Geometry check sheet. Reference: the model listing, model coordinates, mm. A direction names the side the tool comes from. Give positions to 0.01 mm unless a question says otherwise; leave off trailing zeros. Write each loop counter-clockwise with the first axis right and the second up, starting at its lowest first coordinate (ties: lowest second). Pieces come first, ordered by that corner, then holes. Notation, with made-up numbers: (18.25, 16) - (34.25, 16) arc R29 ccw to (34.25, 54) - close; hole circle Ø8 at (58.25, -21.75). An arc over 180 degrees is marked (long way). One line per question, with ' | ' between items. Start each with the question number.
Q1. Set-up check for faces 1 (the face through (-118.726, 56.298, 153.37)), 2 (the face through (152.4, -95, -28)), 3 (the face through (101.6, -1, -64)): record each of +Z, -Z, +X, -X, +Y, -Y from which the full face is reachable in a straight line by a thin tool's end or side.
Q2. Section check B-B on z = -25.4. Record the boundary of the cut face in (x, y), and give its area (3 significant figures).
Q3. Section check C-C on x = 18. Record the boundary of the cut face in (y, z).
Q4. Release check for a two-part mould opening along X. For faces 4 (the face through (1.355, 120.166, -156.446)), 5 (the face through (-152.4, -46, -28)), 6 (the face through (118.726, 56.298, 153.37)), 7 (the face through (-23.622, -8.259, -62.594)) record: +X half, -X half, draft (parallel to the pull), parting line (faces both ways), or undercut.
Q5. Section check A-A on y = 0. Record the boundary of the cut face in (x, z).
Q6. Gauge pin test, flat ends, axial feed: P1, Ø2, axis at x = -110, z = -52, coming from the +Y side; P2, Ø5, axis at x = -121, y = -148, coming from the -Z side; P3, Ø1, axis at x = -95.5, y = 139.5, coming from the +Z side. Record the tip position at first contact, or that the pin passes through.
Q7. Thickness scan on L1, parallel to Y at x = 16.5, z = -26; L2, parallel to Z at x = 142.5, y = 0; L3, parallel to X at y = -202.5, z = -77.5. Record the ranges inside material, lowest first. Write a range as [from, to].
```python
from build123d import *

# Parameters (mm, degrees)
F3_R     = 38.1
F3_R_2   = 25.4
F4_DEPTH = 304.801
F5_R     = 88.9
F5_R_2   = 38.1
F6_DEPTH = 50.8


with BuildPart() as f1:
    # F0 (on Front) → F1 (revolve)
    with BuildSketch(Plane.XZ):
        with BuildLine():
            Line((-152.4, 0), (0, 0))
            Line((0, 0), (0, 152.4))
            Line((0, 152.4), (-96.757379, 152.4))
            ThreePointArc((-96.757379, 152.4), (-107.418768, 153.949285), (-116.478976, 159.778363))
            Line((-116.478976, 159.778363), (-152.4, 195.699387))
            Line((-152.4, 195.699387), (-152.4, 0))
        make_face()
    revolve(axis=Axis((-127.974883, 0, -25.4), (-1, 0, 0)))

    # F2: F1 across face


with BuildPart() as f1_1:
    add(f1.part)
    add(f1.part.mirror(Plane(origin=(0, 0, -25.4), x_dir=(0, 1, 0), z_dir=(1, 0, 0))))

    # F3 (on face) → F4 (cut, through all)
    with BuildSketch(Plane.YZ.offset(152.4)):
        with Locations((0, -25.4)):
            Circle(F3_R)
        with Locations((0, -25.4)):
            Circle(F3_R_2, mode=Mode.SUBTRACT)
    extrude(amount=-F4_DEPTH, mode=Mode.SUBTRACT)

    # F5 (on face) → F6 (cut)
    with BuildSketch(Plane.YZ.offset(152.4)):
        with Locations((0, -25.4)):
            Circle(F5_R)
        with Locations((0, -25.4)):
            Circle(F5_R_2, mode=Mode.SUBTRACT)
    extrude(amount=-F6_DEPTH, mode=Mode.SUBTRACT)


solid = f1_1.part
```
Working result:
1) face 1: none | face 2: +Z, -Z, +X, +Y, -Y | face 3: +X
2) outline: (-152.4, -221.1) - (-116.48, -185.18) arc R25.4 cw to (-96.76, -177.8) - (96.76, -177.8) arc R25.4 cw to (116.48, -185.18) - (152.4, -221.1) - (152.4, -88.9) - (101.6, -88.9) - (101.6, -38.1) - (-152.4, -38.1) - close; (-152.4, 38.1) - (101.6, 38.1) - (101.6, 88.9) - (152.4, 88.9) - (152.4, 221.1) - (116.48, 185.18) arc R25.4 cw to (96.76, 177.8) - (-96.76, 177.8) arc R25.4 cw to (-116.48, 185.18) - (-152.4, 221.1) - close | area: 83,800 mm2
3) outline: circle Ø355.6 at (0, -25.4); hole circle Ø76.2 at (0, -25.4)
4) face 4: undercut | face 5: -X half | face 6: undercut | face 7: draft
5) outline: (-152.4, -246.5) - (-116.48, -210.58) arc R25.4 cw to (-96.76, -203.2) - (96.76, -203.2) arc R25.4 cw to (116.48, -210.58) - (152.4, -246.5) - (152.4, -114.3) - (101.6, -114.3) - (101.6, -63.5) - (-152.4, -63.5) - close; (-152.4, 12.7) - (101.6, 12.7) - (101.6, 63.5) - (152.4, 63.5) - (152.4, 195.7) - (116.48, 159.78) arc R25.4 cw to (96.76, 152.4) - (-96.76, 152.4) arc R25.4 cw to (-116.48, 159.78) - (-152.4, 195.7) - close
6) P1: stops at y = 179.07 | P2: stops at z = -149.04 | P3: stops at z = 85.47
7) L1: y = [-177.8, -38.1], [38.1, 177.8] | L2: z = [-236.6, -114.3], [63.5, 185.8] | L3: x = [-152.4, -140.4], [140.4, 152.4]
